The model under review builds one solid part; all positions refer to its coordinate system, in mm. Face numbers are marked on the shaded views. Coordinates: 2 decimals unless noted, no trailing zeros. Loops run counter-clockwise (first coordinate to the right, second up) from the corner with the lowest first, then second, coordinate; pieces in that order, holes last. Notation, with made-up numbers: (23.5, -2.75) - (35.5, -2.75) arc R31 ccw to (35.5, 25.25) - close; hole circle Ø10 at (-9.5, 1). An arc over 180 degrees is marked (long way). Use a Markdown table: item, result. Add a question column.
1) Add section A-A, the plane x = 0. Give the boundary of the cut face in (y, z).
2) Add section C-C, the plane y = 0.4. Give the boundary of the cut face in (x, z).
3) Clearance check with flat-ended pins moving along their axes: pin 1 (4 mm diameter, centred on x = 5.5, z = -4, fed in from -Y); pin 2 (1.5 mm diameter, centred on y = 1, z = 2.5, fed in from -X); pin 3 (10 mm diameter, centred on x = 0, z = 0, fed in from -Y). State where each tip first meets the part, or that it passes through.
4) To check wall thickness, follow L1, parallel to X at y = 3.15, z = 0; L2, parallel to X at y = 1.3, z = 1.25. State the ranges of each line that lie inside material, in increasing order. Write a range as [from, to].
5) Add section B-B, the plane z = -5. Give the boundary of the cut face in (x, y).
6) The part is to be moulded in two halves that separate along X. For the marked faces 1, 2 and 3, say which applies: pulls with the +X half, pulls with the -X half, needs draft (parallel to the pull), parting line crosses it, or undercut.
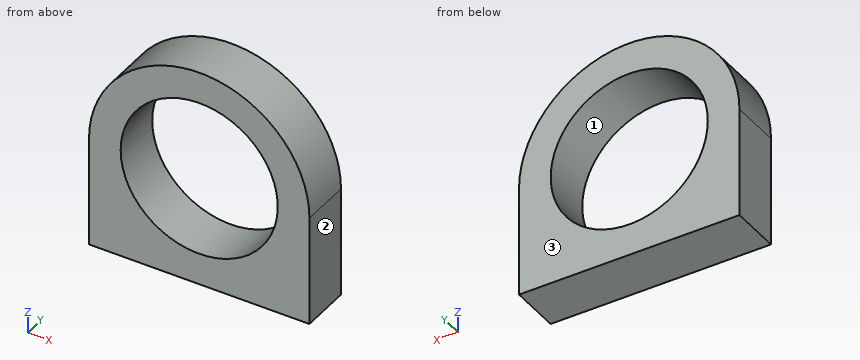
Autodesk Inventor part; units mm, degrees
ref_plane "YZ Plane" through (0, 0, 0) normal (1, 0, 0) x (0, 1, 0)
ref_plane "XZ Plane" through (0, 0, 0) normal (0, 1, 0) x (-1, 0, 0)
ref_plane "XY Plane" through (0, 0, 0) normal (0, 0, 1) x (1, 0, 0)
sketch "Sketch1" plane through (0, 0, 0) normal (0, 1, 0) x (-1, 0, 0)
  circle A0 centre (0, 0) radius 2
  circle A1 centre (0, 0) radius 6.2
  circle A2 centre (0, 0) radius 8.7
  line L0 (12.18, 0) -> (-12.18, 0)
  line L1 (0, -12.18) -> (0, 12.18)
  line L2 (8.7, 0) -> (8.7, -8.7)
  line L3 (8.7, -8.7) -> (-8.7, -8.7)
  line L4 (-8.7, -8.7) -> (-8.7, 0)
  dimension "d0" = 4
  dimension "d1" = 12.4
  dimension "d2" = 17.4
  dimension "d3" = 17.4
extrude "Extrusion1" add sketch "Sketch1" along normal blind 4 contours L0 A2 L1 A1 | A1 L1 A2 L0 | A1 L0 A2 L1 | L1 A2 L0 A1 | L2 L3 A2 | L3 L4 A2
properties part number "borde al borde chico"
From the geometry:
| question | item | result |
|---|---|---|
| 1 | outline | (0, -8.7) - (4, -8.7) - (4, -6.2) - (0, -6.2) - close; (0, 6.2) - (4, 6.2) - (4, 8.7) - (0, 8.7) - close |
| 2 | outline | (-8.7, -8.7) - (8.7, -8.7) - (8.7, 0) arc R8.7 ccw to (-8.7, 0) - close; hole circle Ø12.4 at (0, 0) |
| 3 | pin 1 | stops at y = 0 |
| 3 | pin 2 | stops at x = -8.52 |
| 3 | pin 3 | passes through |
| 4 | L1 | x = [-8.7, -6.2], [6.2, 8.7] |
| 4 | L2 | x = [-8.61, -6.07], [6.07, 8.61] |
| 5 | outline | (-8.7, 0) - (-3.67, 0) - (-3.67, 4) - (-8.7, 4) - close; (3.67, 0) - (8.7, 0) - (8.7, 4) - (3.67, 4) - close |
| 6 | face 1 | undercut |
| 6 | face 2 | pulls with the +X half |
| 6 | face 3 | needs draft |
